Design review of the part built by this model. Coordinates are the model's own, in mm. Face numbers are marked on the shaded views. A direction names the side the tool comes from. Give positions to 0.01 mm unless a question says otherwise; leave off trailing zeros. Write each loop counter-clockwise with the first axis right and the second up, starting at its lowest first coordinate (ties: lowest second). Pieces come first, ordered by that corner, then holes.
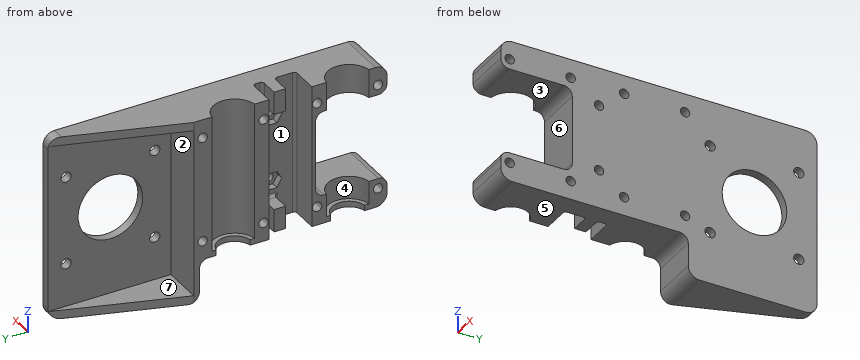
```python
from build123d import *

# Parameters (mm, degrees)
SKETCH1_W               = 7
SKETCH1_H               = 67.54
BOSS_EXTRUDE1_DEPTH     = 50
SKETCH2_W               = 50
SKETCH2_H               = 26.27
BOSS_EXTRUDE2_DEPTH     = 10
SKETCH3_R               = 7.5
CUT_EXTRUDE1_DEPTH      = 62.827687164
SKETCH4_W               = 100
SKETCH4_H               = 30
CUT_EXTRUDE2_DEPTH      = 25
BOSS_EXTRUDE3_START     = -2
BOSS_EXTRUDE3_DEPTH     = 2
CUT_EXTRUDE3_DEPTH      = 63.685029313
CUT_EXTRUDE3_DEPTH_BACK = 63.685029313
SKETCH6_R               = 1.65
SKETCH7_W               = 65
SKETCH7_H               = 43
BOSS_EXTRUDE4_DEPTH     = 3
CUT_EXTRUDE4_DEPTH      = 94.180646596
CUT_EXTRUDE4_DEPTH_BACK = 94.180646596
SKETCH8_R               = 1.8
SKETCH8_R_2             = 11.3
CUT_EXTRUDE5_DEPTH      = 94.180646596
CUT_EXTRUDE5_DEPTH_BACK = 94.180646596
SKETCH11_R              = 1.65
SKETCH12_W              = 8
SKETCH12_H              = 4
BOSS_EXTRUDE6_DEPTH     = 7
SKETCH15_W              = 17
SKETCH15_H              = 15
BOSS_EXTRUDE7_DEPTH     = 2
FILLET4_R               = 3
FILLET5_R               = 3
FILLET6_R               = 1
BOSS_EXTRUDE8_DEPTH     = 3
BOSS_EXTRUDE9_DEPTH     = 3
FILLET7_R               = 4
CUT_EXTRUDE7_DEPTH      = 2.5


with BuildPart() as part:
    # Sketch1 → Boss-Extrude1 (new body)
    with BuildSketch(Plane.XY):
        Rectangle(SKETCH1_W, SKETCH1_H)
    extrude(amount=BOSS_EXTRUDE1_DEPTH)

    # Sketch2 → Boss-Extrude2 (add)
    with BuildSketch(Plane.ZY.offset(3.5)):
        with Locations((25, 20.635)):
            Rectangle(SKETCH2_W, SKETCH2_H)
        with Locations((25, -20.635)):
            Rectangle(SKETCH2_W, SKETCH2_H)
    extrude(amount=BOSS_EXTRUDE2_DEPTH)

    # Sketch3 → Cut-Extrude1 (cut, through all)
    with BuildSketch(Plane.XY.offset(50)):
        with Locations((-14.5, 20)):
            Circle(SKETCH3_R)
        with Locations((-14.5, -20)):
            Circle(SKETCH3_R)
    extrude(amount=-CUT_EXTRUDE1_DEPTH, mode=Mode.SUBTRACT)

    # Sketch4 → Cut-Extrude2 (cut)
    with BuildSketch(Plane.XZ.offset(33.77)):
        with Locations((13.05, 25)):
            Rectangle(SKETCH4_W, SKETCH4_H)
    extrude(amount=-CUT_EXTRUDE2_DEPTH, mode=Mode.SUBTRACT)

    # Sketch5 → Boss-Extrude3 (add)
    with BuildSketch(Plane(origin=(0, 0, 0), x_dir=(-1, 0, 0), z_dir=(0, 0, -1)).offset(BOSS_EXTRUDE3_START)):
        with BuildLine():
            Line((13.5, 27.433034374), (13.5, 25.916079783))
            ThreePointArc((13.5, 25.916079783), (8.5, 20), (13.5, 14.083920217))
            Line((13.5, 14.083920217), (13.5, 12.566965626))
            ThreePointArc((13.5, 12.566965626), (7, 20), (13.5, 27.433034374))
        make_face()
        with BuildLine():
            Line((13.5, -12.566965626), (13.5, -14.083920217))
            ThreePointArc((13.5, -14.083920217), (8.5, -20), (13.5, -25.916079783))
            Line((13.5, -25.916079783), (13.5, -27.433034374))
            ThreePointArc((13.5, -27.433034374), (7, -20), (13.5, -12.566965626))
        make_face()
    extrude(amount=BOSS_EXTRUDE3_DEPTH)

    # Sketch6 → Cut-Extrude3 (cut, two sides: drawn at the far end of the back side and taken through both)
    with BuildSketch(Plane(origin=(3.5, 0, 0), x_dir=(0, 0, -1), z_dir=(1, 0, 0)).offset(-CUT_EXTRUDE3_DEPTH_BACK)):
        with Locations(Location((-6.5, 30.65196164, 0), (0, 0, 180))):
            Circle(SKETCH6_R)
        with Locations(Location((-6.5, 9.34803836, 0), (0, 0, 180))):
            Circle(SKETCH6_R)
        with Locations(Location((-43.5, 9.34803836, 0), (0, 0, 180))):
            Circle(SKETCH6_R)
        with Locations(Location((-43.5, 30.65196164, 0), (0, 0, 180))):
            Circle(SKETCH6_R)
        with Locations((-43.5, -9.34803836)):
            Circle(SKETCH6_R)
        with Locations((-43.5, -30.65196164)):
            Circle(SKETCH6_R)
        with Locations((-6.5, -9.34803836)):
            Circle(SKETCH6_R)
        with Locations((-6.5, -30.65196164)):
            Circle(SKETCH6_R)
    extrude(amount=CUT_EXTRUDE3_DEPTH + CUT_EXTRUDE3_DEPTH_BACK, mode=Mode.SUBTRACT)

    # Sketch7 → Boss-Extrude4 (add)
    with BuildSketch(Plane(origin=(3.5, 0, 0), x_dir=(0, 0, -1), z_dir=(1, 0, 0))):
        with Locations((-17.5, 55.27)):
            Rectangle(SKETCH7_W, SKETCH7_H)
    extrude(amount=-BOSS_EXTRUDE4_DEPTH)

    # Sketch8 → Cut-Extrude4 (cut, two sides: drawn at the far end of the back side and taken through both)
    with BuildSketch(Plane(origin=(3.5, 0, 0), x_dir=(0, 0, -1), z_dir=(1, 0, 0)).offset(-CUT_EXTRUDE4_DEPTH_BACK)):
        with Locations(Location((-3.15, 70.42, 0), (0, 0, 180))):
            Circle(SKETCH8_R)
        with Locations(Location((-3.15, 39.42, 0), (0, 0, 180))):
            Circle(SKETCH8_R)
        with Locations(Location((-34.15, 70.42, 0), (0, 0, 180))):
            Circle(SKETCH8_R)
        with Locations(Location((-18.65, 54.92, 0), (0, 0, 180))):
            Circle(SKETCH8_R_2)
        with Locations(Location((-34.15, 39.42, 0), (0, 0, 180))):
            Circle(SKETCH8_R)
    extrude(amount=CUT_EXTRUDE4_DEPTH + CUT_EXTRUDE4_DEPTH_BACK, mode=Mode.SUBTRACT)

    # Sketch11 → Cut-Extrude5 (cut, two sides: drawn at the far end of the back side and taken through both)
    with BuildSketch(Plane(origin=(3.5, 0, 0), x_dir=(0, 0, -1), z_dir=(1, 0, 0)).offset(-CUT_EXTRUDE5_DEPTH_BACK)):
        with Locations((-36.590767043, 0.58)):
            Circle(SKETCH11_R)
        with Locations((-13.409232957, 0.58)):
            Circle(SKETCH11_R)
    extrude(amount=CUT_EXTRUDE5_DEPTH + CUT_EXTRUDE5_DEPTH_BACK, mode=Mode.SUBTRACT)

    # Sketch12 → Boss-Extrude6 (add)
    with BuildSketch(Plane.ZY.offset(3.5)):
        with Locations((4, 2)):
            Rectangle(SKETCH12_W, SKETCH12_H)
        with Locations((46, 2)):
            Rectangle(SKETCH12_W, SKETCH12_H)
    extrude(amount=BOSS_EXTRUDE6_DEPTH)

    # Sketch15 → Boss-Extrude7 (add)
    with BuildSketch(Plane.XZ.offset(-33.77)):
        with Locations((-5, -7.5)):
            Rectangle(SKETCH15_W, SKETCH15_H)
    extrude(amount=BOSS_EXTRUDE7_DEPTH)

    # Fillet4
    fillet4_edges = [part.edges().sort_by_distance(p)[0] for p in [
        (-5, 31.77, 0),
    ]]
    fillet(fillet4_edges, radius=FILLET4_R)

    # Fillet5
    fillet5_edges = [part.edges().sort_by_distance(p)[0] for p in [
        (-5, -33.77, 40),
        (-5, -33.77, 10),
        (-5, -8.77, 40),
        (-5, -8.77, 10),
    ]]
    fillet(fillet5_edges, radius=FILLET5_R)

    # Fillet6
    fillet6_edges = [part.edges().sort_by_distance(p)[0] for p in [
        (-3.5, 2, 8),
        (-3.5, 2, 42),
        (-3.5, 0, 46),
        (-3.5, 4, 46),
        (-3.5, 4, 4),
        (-3.5, 0, 4),
        (-3.5, 7.5, 25),
        (-3.5, -7.5, 25),
    ]]
    fillet(fillet6_edges, radius=FILLET6_R)

    # Sketch17 → Boss-Extrude8 (add)
    with BuildSketch(Plane.XY.offset(50)):
        Polygon((0.5, 76.77), (-13.5, 33.77), (0.5, 33.77), align=None)
    extrude(amount=-BOSS_EXTRUDE8_DEPTH)

    # Sketch18 → Boss-Extrude9 (add)
    with BuildSketch(Plane(origin=(0, 0, -15), x_dir=(-1, 0, 0), z_dir=(0, 0, -1))):
        Polygon((-0.5, 76.77), (13.5, 33.77), (-0.5, 33.77), align=None)
    extrude(amount=-BOSS_EXTRUDE9_DEPTH)

    # Fillet7
    # the kernel refuses this fillet: 4 mm, written as the material it takes off along each edge
    with BuildSketch(Plane(origin=(13.5, -33.77, 50), x_dir=(0, 1, 0), z_dir=(-1, 0, 0)), Plane(origin=(-23.5, -33.77, 0), x_dir=(0, 1, 0), z_dir=(1, 0, 0)), Plane(origin=(13.5, 31.77, -15), x_dir=(0, 0, 1), z_dir=(-1, 0, 0))) as fillet7_piece_1:
        with BuildLine():
            CenterArc((FILLET7_R, FILLET7_R), FILLET7_R, 180, 90)
            Line((0, FILLET7_R), (0, 0))
            Line((0, 0), (FILLET7_R, 0))
        make_face()
    extrude(amount=37, mode=Mode.SUBTRACT)
    with BuildSketch(Plane(origin=(13.5, 76.77, -15), x_dir=(0, -1, 0), z_dir=(-1, 0, 0))) as fillet7_piece_2:
        with BuildLine():
            CenterArc((FILLET7_R, FILLET7_R), FILLET7_R, 180, 90)
            Line((0, FILLET7_R), (0, 0))
            Line((0, 0), (FILLET7_R, 0))
        make_face()
    extrude(amount=23, mode=Mode.SUBTRACT)
    with BuildSketch(Plane(origin=(13.5, 76.77, 50), x_dir=(0, -1, 0), z_dir=(-1, 0, 0))) as fillet7_piece_3:
        with BuildLine():
            CenterArc((FILLET7_R, -FILLET7_R), FILLET7_R, 90, 90)
            Line((0, -FILLET7_R), (0, 0))
            Line((0, 0), (FILLET7_R, 0))
        make_face()
    extrude(amount=23, mode=Mode.SUBTRACT)

    # Sketch19 → Cut-Extrude7 (cut)
    with BuildSketch(Plane.ZY.offset(3.5)):
        Polygon((13.409232957, 3.870896534), (10.559232957, 2.225448267), (10.559232957, -1.065448267), (13.409232957, -2.710896534), (16.259232957, -1.065448267), (16.259232957, 2.225448267), align=None)
        Polygon((36.590767043, 3.870896534), (33.740767043, 2.225448267), (33.740767043, -1.065448267), (36.590767043, -2.710896534), (39.440767043, -1.065448267), (39.440767043, 2.225448267), align=None)
    extrude(amount=-CUT_EXTRUDE7_DEPTH, mode=Mode.SUBTRACT)


solid = part.part
```
(1) Mouldability with a two-part tool opening along Y and no side actions: class the marked faces 1, 2 and 3 as pulls with the +Y half, pulls with the -Y half, needs draft (parallel to the pull), parting line crosses it, or undercut.
Resolved:
face 1: undercut
face 2: pulls with the +Y half
face 3: needs draft
(2) Consider section B-B, the plane y = 70.42. Give the boundary of the cut face in (x, z).
Resolved:
outline: (-1.57, -15) - (3.5, -15) - (3.5, 1.35) - (0.5, 1.35) - (0.5, -12) - (-1.57, -12) - close; (-1.57, 47) - (0.5, 47) - (0.5, 35.95) - (3.5, 35.95) - (3.5, 50) - (-1.57, 50) - close; (0.5, 4.95) - (3.5, 4.95) - (3.5, 32.35) - (0.5, 32.35) - close
(3) Tool access review of the marked faces 4, 5, 6 and 7: name each direction out of +Z, -Z, +X, -X, +Y, -Y from which nothing blocks a thin tool from reaching the whole face with its end or side.
Resolved:
face 4: +Z, -X
face 5: -Z, +X, -X, -Y
face 6: +X, -X, -Y
face 7: -X, +Y
(4) Consider section C-C, the plane y = -24. Give the boundary of the cut face in (x, z).
Resolved:
outline: (-10.03, 0) - (3.5, 0) - (3.5, 10) - (-8.16, 10) - (-8.16, 2) - (-10.03, 2) - close; (-8.16, 40) - (3.5, 40) - (3.5, 50) - (-8.16, 50) - close
(5) Consider section A-A, the plane z = 18.65. Give the boundary of the cut face in (x, y), then the cut area to 3 significant figures.
Resolved:
outline: (-13.5, -8.77) - (3.5, -8.77) - (3.5, 43.62) - (0.5, 43.62) - (0.5, 33.77) - (-13.5, 33.77) - (-13.5, 27.43) arc R7.5 cw to (-13.5, 12.57) - (-13.5, 7.5) - (-4.5, 7.5) arc R1 cw to (-3.5, 6.5) - (-3.5, -6.5) arc R1 cw to (-4.5, -7.5) - (-13.5, -7.5) - close; (0.5, 66.22) - (3.5, 66.22) - (3.5, 76.77) - (0.5, 76.77) - close
area: 561 mm2
(6) To check wall thickness, follow L1, parallel to Y at x = -1, z = 43.5; L2, parallel to Z at x = 0.15, y = 0.58; L3, parallel to Z at x = 0, y = 70. State the ranges of each line that lie inside material, in increasing order.
Resolved:
L1: y = -33.77 to -32.3, -29 to -11, -7.7 to 7.7, 11 to 29, 32.3 to 33.77
L2: z = 0 to 11.76, 15.06 to 34.94, 38.24 to 50
L3: z = -15 to -12, 47 to 50
(7) Consider section D-D, the plane z = -4.5. Give the boundary of the cut face in (x, y), then the cut area to 3 significant figures.
Resolved:
outline: (-13.5, 31.77) - (3.5, 31.77) - (3.5, 76.77) - (0.5, 76.77) - (0.5, 33.77) - (-13.5, 33.77) - close
area: 163 mm2
(8) Clearance check with flat-ended pins moving along their axes: P1, Ø2.5, axis at y = 9.35, z = 43.5, coming from the -X side; P2, Ø6, axis at x = -6.5, y = 21, coming from the -Z side; P3, Ø1.2, axis at y = 1.5, z = 45, coming from the -X side; P4, Ø13, axis at y = 60, z = 25.5, coming from the -X side. State where each tip first meets the part, or that it passes through.
Resolved:
P1: passes through
P2: stops at z = 0
P3: stops at x = -10.5
P4: stops at x = 0.5
